from build123d import *

# Parameters (mm, degrees)
F0_R     = 20
F0_R_2   = 16
F0_R_3   = 30
F1_DEPTH = 30


with BuildPart() as f1:
    # F0 (on Front) → F1 (new body)
    with BuildSketch(Plane.XZ):
        with BuildLine():
            Line((57.179358, 216.494742), (-60.600481, 216.494742))
            Line((-60.600481, 216.494742), (-60.600481, -63.505258))
            Line((-60.600481, -63.505258), (7.520599, -63.505258))
            Line((7.520599, -63.505258), (58.176437, -63.505258))
            Line((58.176437, -63.505258), (61.640235, -63.505258))
            ThreePointArc((61.640235, -63.505258), (27.911346, -44.351415), (14.340876, -8.014795))
            Line((14.340876, -8.014795), (12.77445, 166.592886))
            ThreePointArc((12.77445, 166.592886), (12.473491, 171.386014), (12.68841, 176.18377))
            ThreePointArc((12.68841, 176.18377), (27.160951, 204.918189), (57.179358, 216.494742))
        make_face()
        with BuildLine():
            ThreePointArc((98.646262, 188.498488), (82.195824, 208.840441), (57.179358, 216.494742))
            ThreePointArc((57.179358, 216.494742), (27.160951, 204.918189), (12.68841, 176.18377))
            Line((12.68841, 176.18377), (12.77445, 166.592886))
            Line((12.77445, 166.592886), (14.340876, -8.014795))
            ThreePointArc((14.340876, -8.014795), (27.911346, -44.351415), (61.640235, -63.505258))
            Line((61.640235, -63.505258), (80.636496, -63.505258))
            Line((80.636496, -63.505258), (132.381109, -63.505258))
            ThreePointArc((132.381109, -63.505258), (168.001141, -36.462478), (170.434949, 8.193711))
            Line((170.434949, 8.193711), (99.25581, 186.898251))
            Line((99.25581, 186.898251), (98.646262, 188.498488))
        make_face()
        with Locations((71.138366, -7.505258)):
            Circle(F0_R, mode=Mode.SUBTRACT)
        with Locations((120.978109, -11.505258)):
            Circle(F0_R_2, mode=Mode.SUBTRACT)
        with Locations((57.179358, 171.787076)):
            Circle(F0_R_3, mode=Mode.SUBTRACT)
        with BuildLine():
            ThreePointArc((99.25581, 186.898251), (98.958698, 187.701288), (98.646262, 188.498488))
            Line((98.646262, 188.498488), (99.25581, 186.898251))
        make_face()
        with BuildLine():
            Line((80.636496, -63.505258), (61.640235, -63.505258))
            ThreePointArc((61.640235, -63.505258), (71.138366, -64.305033), (80.636496, -63.505258))
        make_face()
    extrude(amount=F1_DEPTH)


solid = f1.part
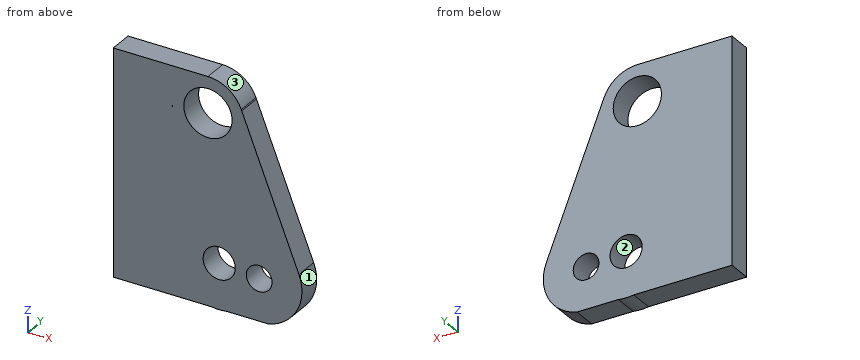
Source: CAD feature listing. Evaluate the final solid. Frame: model axes, mm. Face numbers are marked on the shaded views. Round coordinates to 2 decimals unless told otherwise and drop trailing zeros. Order: outer loops, then holes, each group sorted by start corner. A loop starts at its lowest first (then second) coordinate and runs counter-clockwise, first axis right, second up. Notation, with made-up numbers: (25.25, -22) - (56.25, -22) arc R13 cw to (56.25, -18) - close; hole circle Ø2 at (-18.5, 69). An arc over 180 degrees is marked (long way). Use a Markdown table: item, result. Add a question column.
1. First-contact query: pin 1 (1.5 mm diameter, centred on x = 67.5, y = -15, fed in from -Z); pin 2 (3 mm diameter, centred on x = -13.5, y = -6.5, fed in from -Z); pin 3 (1.5 mm diameter, centred on y = -20, z = 29, fed in from +X). Flat tips, straight axial feed; report the tip coordinate or a pass-through.
2. Line query: probe 1 along Z at (x, y) = (71.5, -1.5); probe 2 along Z at (x, y) = (63, -7.25); probe 3 along X at (y, z) = (-11.5, -13.5). Output: solid intervals per line, ascending.
3. Section query D-D (y = -9.75). Return the cut outline in (x, z).
4. Section query C-C (x = 66). Return the cut outline in (y, z).
5. Mould query, pull axis Z, two halves, no side actions, for the marked faces 1, 2 and 3. Classes: +Z half, -Z half, draft (parallel to the pull), parting line (faces both ways), or undercut.
6. Section query B-B (z = 149). Return the cut outline in (x, y), then the cut area to 3 significant figures.
7. Section query A-A (x = 42.5). Return the cut outline in (y, z).
Derived:
| question | item | result |
|---|---|---|
| 1 | pin 1 | z = -64.23 |
| 1 | pin 2 | z = -63.51 |
| 1 | pin 3 | x = 162.45 |
| 2 | probe 1 | -64.3 to -27.5, 12.49 to 145.43, 198.15 to 214.14 |
| 2 | probe 2 | -63.72 to -25.77, 10.76 to 142.36, 201.22 to 216.11 |
| 2 | probe 3 | -60.6 to 52.06, 90.22 to 105.1, 136.85 to 174.18 |
| 3 | outline | (-60.6, -63.51) - (61.64, -63.51) arc R56.8 ccw to (80.64, -63.51) - (132.38, -63.51) arc R53.24 ccw to (170.43, 8.19) - (99.26, 186.9) arc R44.71 ccw to (98.65, 188.5) arc R44.71 ccw to (57.18, 216.49) - (-60.6, 216.49) - close; hole (12.69, 176.18) arc R44.71 ccw to (12.77, 166.59) - close; hole circle Ø60 at (57.18, 171.79); hole circle Ø40 at (71.14, -7.51); hole circle Ø32 at (120.98, -11.51) |
| 4 | outline | (-30, -64.07) - (0, -64.07) - (0, -26.83) - (-30, -26.83) - close; (-30, 11.82) - (0, 11.82) - (0, 143.11) - (-30, 143.11) - close; (-30, 200.46) - (0, 200.46) - (0, 215.62) - (-30, 215.62) - close |
| 5 | face 1 | parting line |
| 5 | face 2 | undercut |
| 5 | face 3 | +Z half |
| 6 | outline | (-60.6, -30) - (37.67, -30) - (37.67, 0) - (-60.6, 0) - close; (76.69, -30) - (114.35, -30) - (114.35, 0) - (76.69, 0) - close |
| 6 | area | 4,080 mm2 |
| 7 | outline | (-30, -63.51) - (0, -63.51) - (0, 145.62) - (-30, 145.62) - close; (-30, 197.95) - (0, 197.95) - (0, 216.49) - (-30, 216.49) - close |
